Design review of the part built by this model. Coordinates are the model's own, in mm. Face numbers are marked on the shaded views. A direction names the side the tool comes from. Round coordinates to 2 decimals unless told otherwise and drop trailing zeros. Order: outer loops, then holes, each group sorted by start corner. A loop starts at its lowest first (then second) coordinate and runs counter-clockwise, first axis right, second up.
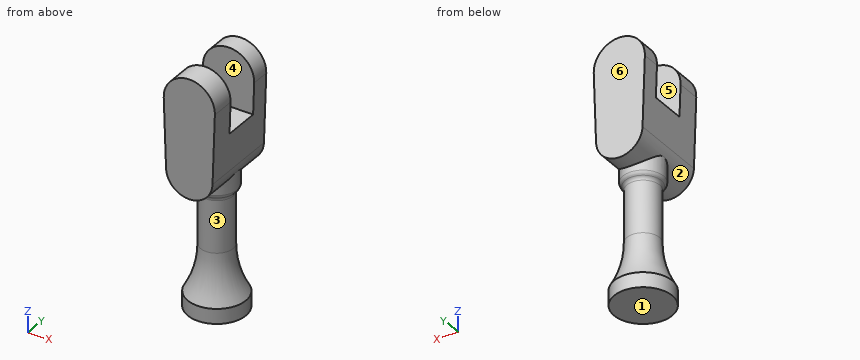
from build123d import *

# Parameters (mm, degrees)
SKETCH_1_R               = 62.5
EXTRUDE_1_DEPTH          = 32
EXTRUDE_2_DEPTH          = 79
EXTRUDE_2_DEPTH_BACK     = 91
CUT_EXTRUDE_1_DEPTH      = 541.396382314
CUT_EXTRUDE_1_DEPTH_BACK = 541.396382314
SKETCH_12_W              = 78
SKETCH_12_H              = 125


with BuildPart() as part:
    # 草圖1 → 填料-伸長1 (new body)
    with BuildSketch(Plane.XY):
        Circle(SKETCH_1_R)
    extrude(amount=EXTRUDE_1_DEPTH)

    # 草圖3 → 旋轉1 (revolve)
    with BuildSketch(Plane(origin=(0, 0, 0), x_dir=(1, 0, 0), z_dir=(0, 1, 0)), mode=Mode.PRIVATE) as revolve_1_sk:
        with BuildLine():
            Line((0, -32), (0, -245))
            Line((0, -245), (35, -245))
            Line((35, -245), (35, -133.211))
            ThreePointArc((35, -133.211), (41.997410306, -80.770756577), (62.5, -32))
            Line((62.5, -32), (0, -32))
        make_face()
    revolve(revolve_1_sk.sketch.rotate(Axis((0, 0, 32), (0, 0, 1)), 180), axis=Axis((0, 0, 32), (0, 0, 1)))

    # 草圖6 → 旋轉2 (revolve)
    with BuildSketch(Plane(origin=(0, 0, 0), x_dir=(1, 0, 0), z_dir=(0, 1, 0))):
        with BuildLine():
            Line((0, -245), (35, -245))
            ThreePointArc((35, -245), (36.015734709, -249.478225638), (38.864145372, -253.08))
            ThreePointArc((38.864145372, -253.08), (41.946904934, -256.68505084), (43.52, -261.16))
            Line((43.52, -261.16), (0, -261.16))
            Line((0, -261.16), (0, -245))
        make_face()
    revolve(axis=Axis((0, 0, 211.16), (0, 0, -1)))

    # 草圖9 → 旋轉3 (revolve)
    with BuildSketch(Plane(origin=(0, 0, 0), x_dir=(1, 0, 0), z_dir=(0, 1, 0)), mode=Mode.PRIVATE) as revolve_3_sk:
        with BuildLine():
            Line((0, -261.16), (0, -322.34))
            Line((0, -322.34), (46.183269827, -322.34))
            ThreePointArc((46.183269827, -322.34), (44.034639015, -291.785565226), (43.52, -261.16))
            Line((43.52, -261.16), (0, -261.16))
        make_face()
    revolve(revolve_3_sk.sketch.rotate(Axis((0, 0, 0), (0, 0, 1)), 180), axis=Axis((0, 0, 0), (0, 0, 1)))

    # 草圖10 → 填料-伸長2 (add, two sides: drawn at the far end of the back side and taken through both)
    with BuildSketch(Plane(origin=(0, 0, 0), x_dir=(0, 0, -1), z_dir=(0, 1, 0)).offset(-EXTRUDE_2_DEPTH_BACK)):
        with BuildLine():
            Line((-322.333333333, 49.972214502), (-472.166666667, 54.969435952))
            ThreePointArc((-472.166666667, 54.969435952), (-529, 0), (-472.166666667, -54.969435952))
            Line((-472.166666667, -54.969435952), (-322.333333333, -49.972214502))
            ThreePointArc((-322.333333333, -49.972214502), (-274, 0), (-322.333333333, 49.972214502))
        make_face()
    extrude(amount=EXTRUDE_2_DEPTH + EXTRUDE_2_DEPTH_BACK)

    # 草圖12 → 除料-伸長1 (cut, two sides: drawn at the far end of the back side and taken through both)
    with BuildSketch(Plane(origin=(0, 0, 0), x_dir=(0, -1, 0), z_dir=(1, 0, 0)).offset(-CUT_EXTRUDE_1_DEPTH_BACK)):
        with Locations((0, -466.5)):
            Rectangle(SKETCH_12_W, SKETCH_12_H)
    extrude(amount=CUT_EXTRUDE_1_DEPTH + CUT_EXTRUDE_1_DEPTH_BACK, mode=Mode.SUBTRACT)


solid = part.part
1) For the marked faces 1 and 2, list the 3-axis set-ups (+Z, -Z, +X, -X, +Y, -Y) from which the entire face can be reached by the end or side of a thin tool; tool diameter is ignored.
Results:
face 1: -Z, +X, -X, +Y, -Y
face 2: none
2) The part is to be moulded in two halves that separate along Y. For the marked faces 3, 4, 5 and 6, say which applies: released by +Y, released by -Y, zero draft, split by the parting line, or undercut.
Results:
face 3: split by the parting line
face 4: undercut
face 5: undercut
face 6: released by +Y
3) Take a section at C-C on x = 0. Give the boundary of the cut face in (y, z), plus the area to 3 significant figures.
Results:
outline: (-91, 274) - (-43.54, 274) arc R573.63 cw to (-43.52, 261.16) arc R12.91 ccw to (-38.86, 253.08) arc R10.38 cw to (-35, 245) - (-35, 133.21) arc R200 cw to (-62.5, 32) - (-62.5, 0) - (62.5, 0) - (62.5, 32) arc R200 cw to (35, 133.21) - (35, 245) arc R10.38 cw to (38.86, 253.08) arc R12.91 ccw to (43.52, 261.16) arc R573.63 cw to (43.54, 274) - (79, 274) - (79, 529) - (39, 529) - (39, 404) - (-39, 404) - (-39, 529) - (-91, 529) - close
area: 56,700 mm2
4) To check wall thickness, follow line 1 along Y through (x, z) = (-15.5, 447.5); line 2 along Z through (x, y) = (-15, -53); line 3 along Z through (x, y) = (-20.5, -18). State the ranges of each line that lie inside material, in increasing order.
Results:
line 1: y = -91 to -39, 39 to 79
line 2: z = 0 to 45.86, 276.3 to 526.92
line 3: z = 0 to 404
5) Take a section at A-A on y = 0. Give the boundary of the cut face in (x, z), plus the area to 3 significant figures.
Results:
outline: (-62.5, 0) - (62.5, 0) - (62.5, 32) arc R200 cw to (35, 133.21) - (35, 245) arc R10.38 cw to (38.86, 253.08) arc R12.91 ccw to (43.52, 261.16) arc R573.63 cw to (44.53, 301.25) arc R50 ccw to (49.97, 322.33) - (52.7, 404) - (-52.7, 404) - (-49.97, 322.33) arc R50 ccw to (-44.53, 301.25) arc R573.63 cw to (-43.52, 261.16) arc R12.91 ccw to (-38.86, 253.08) arc R10.38 cw to (-35, 245) - (-35, 133.21) arc R200 cw to (-62.5, 32) - close
area: 35,900 mm2
6) Clearance check with flat-ended pins moving along their axes: P1, Ø1.5, axis at y = -67, z = 346.5, coming from the -X side; P2, Ø4, axis at y = 18.5, z = 88.5, coming from the +X side; P3, Ø1.5, axis at x = -28, z = 179.5, coming from the +Y side. State where each tip first meets the part, or that it passes through.
Results:
P1: stops at x = -50.8
P2: stops at x = 36.64
P3: stops at y = 21.96
7) Take a section at B-B on z = 462. Give the boundary of the cut face in (x, y).
Results:
outline: (-54.63, -91) - (54.63, -91) - (54.63, -39) - (-54.63, -39) - close; (-54.63, 39) - (54.63, 39) - (54.63, 79) - (-54.63, 79) - close
8) Take a section at D-D on y = -68.5. Give the boundary of the cut face in (x, z), plus the area to 3 significant figures.
Results:
outline: (-54.97, 472.17) - (-49.97, 322.33) arc R50 ccw to (49.97, 322.33) - (54.97, 472.17) arc R55 ccw (long way) to start
area: 24,400 mm2
